Check sheet for the modelled part. Datum: model origin and axes. Units: mm. Face numbers are marked on the shaded views. A direction names the side the tool comes from. Give positions to 0.01 mm unless a question says otherwise; leave off trailing zeros. Order: outer loops, then holes, each group sorted by start corner. A loop starts at its lowest first (then second) coordinate and runs counter-clockwise, first axis right, second up. Notation, with made-up numbers: (-32, -8) - (-12, -8) arc R34 cw to (-12, 30) - close; hole circle Ø7 at (44.25, -5). An arc over 180 degrees is marked (long way). Answer in a Markdown table with one row per item.
Autodesk Inventor part; units mm, degrees
ref_plane "YZ Plane" through (0, 0, 0) normal (1, 0, 0) x (0, 1, 0)
ref_plane "XZ Plane" through (0, 0, 0) normal (0, 1, 0) x (-1, 0, 0)
ref_plane "XY Plane" through (0, 0, 0) normal (0, 0, 1) x (1, 0, 0)
sketch "スケッチ1" plane through (0, 0, 0) normal (0, 0, 1) x (1, 0, 0)
  line L0 (4.5, -4.5) -> (-4.5, -4.5)
  line L1 (-4.5, -4.5) -> (-4.5, 4.5)
  line L2 (-4.5, 4.5) -> (4.5, 4.5)
  line L3 (4.5, 4.5) -> (4.5, -4.5)
  line L4 (4.5, -4.5) -> (-4.5, 4.5) construction
  line L5 (-4.5, -4.5) -> (4.5, 4.5) construction
  line L6 (3.5, 3.5) -> (-3.5, 3.5)
  line L7 (-3.5, 3.5) -> (-3.5, -3.5)
  line L8 (-3.5, -3.5) -> (3.5, -3.5)
  line L9 (3.5, -3.5) -> (3.5, 3.5)
  point P0 (0, 0)
  dimension "d0" = 9
  dimension "d1" = 9
  dimension "d2" = 1
extrude "押し出し1" add sketch "スケッチ1" along normal blind 30
sketch "スケッチ2" plane through (-4.5, 4.5, 0) normal (0, 1, 0) x (1, 0, 0)
  line L0 (0, 0) -> (9, 0)
  line L1 (0, 0) -> (0, -30)
  line L2 (9, -30) -> (0, -30)
  line L3 (9, 0) -> (9, -30)
  line L4 (4.5, -30) -> (4.5, 0) construction
  line L5 (4.5, -15) -> (0, -15) construction
  circle A0 centre (4.5, -26) radius 1.6
  circle A1 centre (4.5, -4) radius 1.6
  dimension "d5" = 3.2
  dimension "d6" = 4
extrude "押し出し2" cut sketch "スケッチ2" against normal through all contours A0 | A1
sketch "スケッチ3" plane through (4.5, -4.5, 0) normal (1, 0, 0) x (0, 0, -1)
  line L0 (0, 9) -> (0, 0)
  line L1 (0, 9) -> (-30, 9)
  line L2 (-30, 0) -> (-30, 9)
  line L3 (0, 0) -> (-30, 0)
  line L4 (-30, 4.5) -> (0, 4.5) construction
  line L5 (-15, 4.5) -> (-15, 9) construction
  circle A0 centre (-21, 4.5) radius 1.6
  circle A1 centre (-9, 4.5) radius 1.6
  line L6 (-9, 4.5) -> (-21, 4.5)
  line L7 (0, 9) -> (-30, 9)
  dimension "d9" = 3.2
  dimension "d13" = 12
extrude "押し出し3" cut sketch "スケッチ3" against normal through all contours A0 | A1
properties part number "肩ピッチ固定角柱B_9×9" material "アルミニウム 2014-T6"
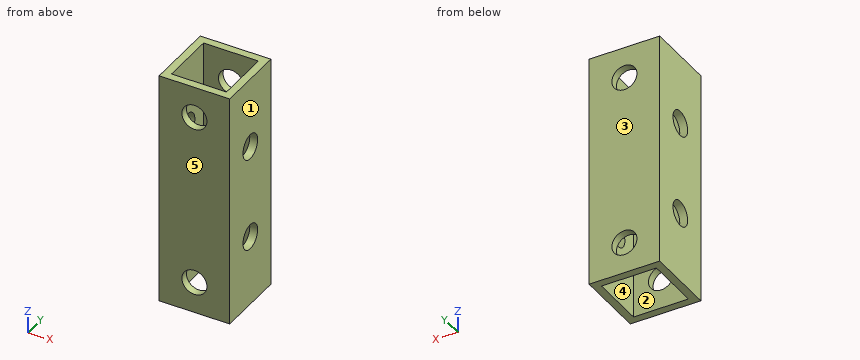
(1) Cross-section at B-B, the plane z = 4. Record the cut outline in (x, y), then the cut area to 3 significant figures.
Geometry says:
| item | result |
|---|---|
| outline | (-4.5, -4.5) - (-1.6, -4.5) - (-1.6, -3.5) - (-3.5, -3.5) - (-3.5, 3.5) - (-1.6, 3.5) - (-1.6, 4.5) - (-4.5, 4.5) - close; (1.6, -4.5) - (4.5, -4.5) - (4.5, 4.5) - (1.6, 4.5) - (1.6, 3.5) - (3.5, 3.5) - (3.5, -3.5) - (1.6, -3.5) - close |
| area | 25.6 mm² |
(2) Gauge pin test, flat end, axial feed: P1, Ø1.5, axis at x = 0, y = -1.5, coming from the -Z side. Record the tip position at first contact, or that the pin passes through.
Geometry says:
| item | result |
|---|---|
| P1 | through |
(3) Cross-section at C-C, the plane y = 2.25. Record the cut outline in (x, z).
Geometry says:
| item | result |
|---|---|
| outline | (-4.5, 0) - (-3.5, 0) - (-3.5, 30) - (-4.5, 30) - close; (3.5, 0) - (4.5, 0) - (4.5, 30) - (3.5, 30) - close |
(4) Thickness scan on L1, parallel to Z at x = 0, y = -3.95; L2, parallel to X at y = -0.5, z = 6.5. Record the ranges inside material, lowest first.
Geometry says:
| item | result |
|---|---|
| L1 | 0 to 2.4, 5.6 to 24.4, 27.6 to 30 |
| L2 | -4.5 to -3.5, 3.5 to 4.5 |
(5) Cross-section at A-A, the plane x = 0. Record the cut outline in (y, z).
Geometry says:
| item | result |
|---|---|
| outline | (-4.5, 0) - (-3.5, 0) - (-3.5, 2.4) - (-4.5, 2.4) - close; (-4.5, 5.6) - (-3.5, 5.6) - (-3.5, 24.4) - (-4.5, 24.4) - close; (-4.5, 27.6) - (-3.5, 27.6) - (-3.5, 30) - (-4.5, 30) - close; (3.5, 0) - (4.5, 0) - (4.5, 2.4) - (3.5, 2.4) - close; (3.5, 5.6) - (4.5, 5.6) - (4.5, 24.4) - (3.5, 24.4) - close; (3.5, 27.6) - (4.5, 27.6) - (4.5, 30) - (3.5, 30) - close |
(6) Mould release check, pull along X, two halves, no side actions. Record for the marked faces 1, 2 and 3: pulls with the +X half, pulls with the -X half, needs draft (parallel to the pull), parting line crosses it, or undercut.
Geometry says:
| item | result |
|---|---|
| face 1 | pulls with the +X half |
| face 2 | undercut |
| face 3 | needs draft |
(7) Access from +Z, -Z, +X, -X, +Y, -Y to the whole of each face (thin tool, end or side, straight path). Record for the marked faces 4 and 5.
Geometry says:
| item | result |
|---|---|
| face 4 | +Z, -Z |
| face 5 | +Z, -Z, +X, -X, -Y |
